from build123d import *

# Parameters (mm, degrees)
SKETCH1_R           = 7.5
BOSS_EXTRUDE1_DEPTH = 2.5
SKETCH2_R           = 29.75
SKETCH2_R_2         = 12
BOSS_EXTRUDE2_DEPTH = 4
SKETCH3_R           = 13.8
BOSS_EXTRUDE3_DEPTH = 26
SKETCH4_R           = 5
CUT_EXTRUDE1_DEPTH  = 25.5
SKETCH5_R           = 2
CUT_EXTRUDE2_DEPTH  = 52.673252268


with BuildPart() as part:
    # Sketch1 → Boss-Extrude1 (new body)
    with BuildSketch(Plane(origin=(0, 0, 0), x_dir=(1, 0, 0), z_dir=(0, 1, 0))):
        with Locations(Location((0, 0, 0), (0, 0, 270))):
            Circle(SKETCH1_R)
    extrude(amount=BOSS_EXTRUDE1_DEPTH)



with BuildPart() as body_2:
    # Sketch2 → Boss-Extrude2 (new body)
    with BuildSketch(Plane.XZ):
        with Locations(Location((0, 0, 0), (0, 0, 270))):
            Circle(SKETCH2_R)
        with Locations(Location((0, 0, 0), (0, 0, 270))):
            Circle(SKETCH2_R_2, mode=Mode.SUBTRACT)
    extrude(amount=-BOSS_EXTRUDE2_DEPTH)


with BuildPart() as part_1:
    add(part.part)

    add(body_2.part)  # Boss-Extrude3 merges body 2
    # Sketch3 → Boss-Extrude3 (add)
    with BuildSketch(Plane.XZ):
        with Locations(Location((0, 0, 0), (0, 0, 90))):
            Circle(SKETCH3_R)
    extrude(amount=BOSS_EXTRUDE3_DEPTH)

    # Sketch4 → Cut-Extrude1 (cut)
    with BuildSketch(Plane.XZ.offset(26)):
        with Locations(Location((0, 0, 0), (0, 0, 270))):
            Circle(SKETCH4_R)
    extrude(amount=-CUT_EXTRUDE1_DEPTH, mode=Mode.SUBTRACT)

    # Sketch5 → Cut-Extrude2 (cut, through all)
    with BuildSketch(Plane(origin=(0, 4, 0), x_dir=(1, 0, 0), z_dir=(0, 1, 0))):
        with Locations(Location((0, 18, 0), (0, 0, 270))):
            Circle(SKETCH5_R)
        with Locations(Location((18, 0, 0), (0, 0, 270))):
            Circle(SKETCH5_R)
        with Locations(Location((0, -18, 0), (0, 0, 270))):
            Circle(SKETCH5_R)
        with Locations(Location((-18, 0, 0), (0, 0, 270))):
            Circle(SKETCH5_R)
    extrude(amount=-CUT_EXTRUDE2_DEPTH, mode=Mode.SUBTRACT)


solid = part_1.part
Geometry check sheet. Reference: the model listing, model coordinates, mm. A direction names the side the tool comes from. Coordinates: 2 decimals unless noted, no trailing zeros. Order: outer loops, then holes, each group sorted by start corner. A loop starts at its lowest first (then second) coordinate and runs counter-clockwise, first axis right, second up. Notation, with made-up numbers: (-3, -40) - (34, -40) arc R22 ccw to (34, -15) - close; hole circle Ø2 at (3, 54.25). An arc over 180 degrees is marked (long way). One line per item, written item: value.
(1) Thickness scan on probe 1 along X at (y, z) = (2.35, 0); probe 2 along X at (y, z) = (2.8, 0); probe 3 along Y at (x, z) = (-4.5, 24). Record the ranges inside material, lowest first. Write a range as from..to.
Data:
probe 1: x = -29.75..-20, -16..-12, -7.5..7.5, 12..16, 20..29.75
probe 2: x = -29.75..-20, -16..-12, 12..16, 20..29.75
probe 3: y = 0..4
(2) Access from +Z, -Z, +X, -X, +Y, -Y to the whole of each face (thin tool, end or side, straight path). Record for faces 1 (the face through (-1.2, 2, 16.4)), 2 (the face through (-4.88, -13.43, 1.08)), 3 (the face through (3.604, 1.972, -11.446)).
Data:
face 1: +Y, -Y
face 2: -Y
face 3: +Y
(3) Sectioned sample at B-B (z = -19). Enter the section's corners in (x, y), and give its area (3 significant figures).
Data:
outline: (-22.89, 0) - (-1.73, 0) - (-1.73, 4) - (-22.89, 4) - close; (1.73, 0) - (22.89, 0) - (22.89, 4) - (1.73, 4) - close
area: 169 mm^2
(4) Depth check by flat-ended pin: pin 1 Ø12 at (x, y) = (-18.5, -18.5) entering from +Z; pin 2 Ø12 at (x, z) = (2.5, 0.5) entering from +Y; pin 3 Ø5 at (x, z) = (-1, 1.5) entering from -Y. Enter the tip coordinate at first touch or a pass-through.
Data:
pin 1: stops at z = 5.85
pin 2: stops at y = 2.5
pin 3: stops at y = -0.5
(5) Release check for a two-part mould opening along X. For faces 4 (the face through (0, 4, -13)), 5 (the face through (-9.33, -12.82, -10.17)), 6 (the face through (0, -0.5, 0)), 7 (the face through (0.33, 1.232, -7.493)) record: +X half, -X half, draft (parallel to the pull), parting line (faces both ways), or undercut.
Data:
face 4: draft
face 5: parting line
face 6: undercut
face 7: undercut
(6) Sectioned sample at D-D (x = 18). Enter the section's corners in (y, z), and give its area (3 significant figures).
Data:
outline: (0, -23.69) - (4, -23.69) - (4, -2) - (0, -2) - close; (0, 2) - (4, 2) - (4, 23.69) - (0, 23.69) - close
area: 173 mm^2
(7) Sectioned sample at C-C (z = -4). Enter the section's corners in (x, y), and give its area (3 significant figures).
Data:
outline: (-29.48, 0) - (-13.21, 0) - (-13.21, -26) - (-3, -26) - (-3, -0.5) - (3, -0.5) - (3, -26) - (13.21, -26) - (13.21, 0) - (29.48, 0) - (29.48, 4) - (11.31, 4) - (11.31, 0) - (6.34, 0) - (6.34, 2.5) - (-6.34, 2.5) - (-6.34, 0) - (-11.31, 0) - (-11.31, 4) - (-29.48, 4) - close
area: 711 mm^2
(8) Sectioned sample at A-A (x = 0). Enter the section's corners in (y, z).
Data:
outline: (-26, -13.8) - (0, -13.8) - (0, -16) - (4, -16) - (4, -12) - (0, -12) - (0, -7.5) - (2.5, -7.5) - (2.5, 7.5) - (0, 7.5) - (0, 12) - (4, 12) - (4, 16) - (0, 16) - (0, 13.8) - (-26, 13.8) - (-26, 5) - (-0.5, 5) - (-0.5, -5) - (-26, -5) - close; (0, -29.75) - (4, -29.75) - (4, -20) - (0, -20) - close; (0, 20) - (4, 20) - (4, 29.75) - (0, 29.75) - close
